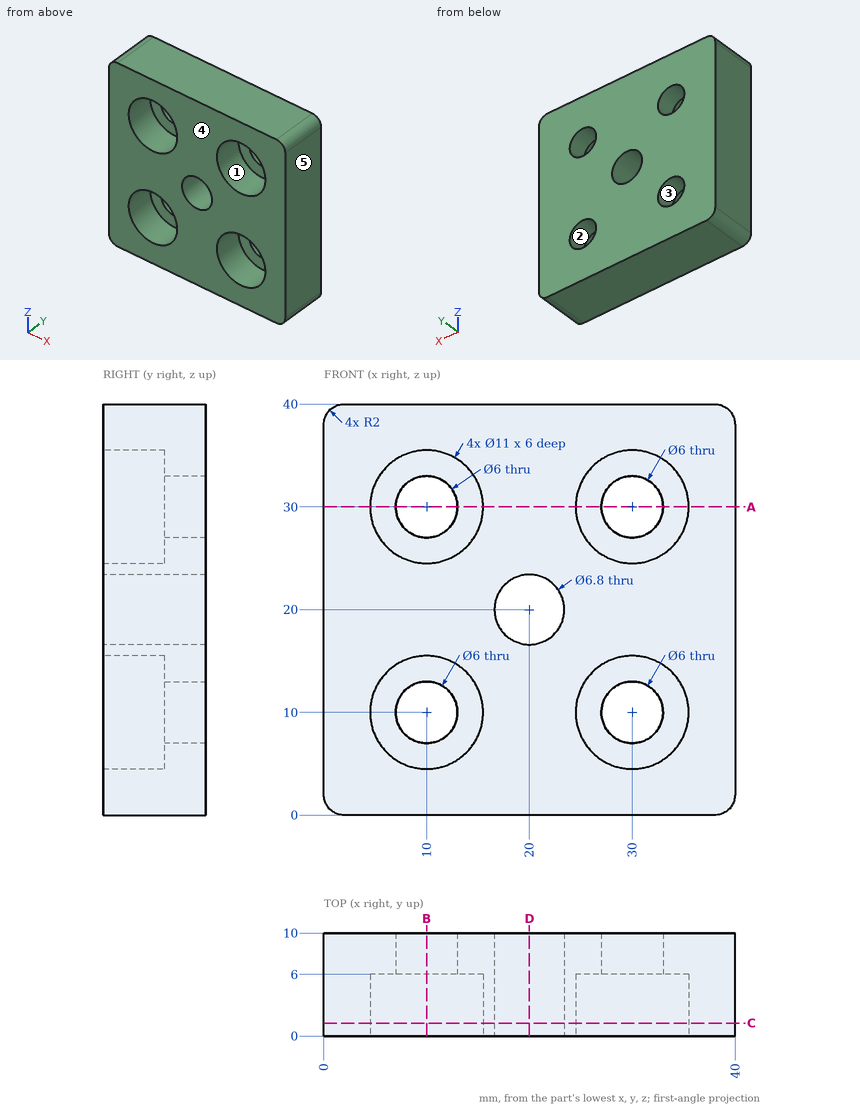
Here's the drawing with two shaded views (mm, measured from the low corner). I have some questions. A direction names the side the tool comes from. Give positions to 0.01 mm unless a question says otherwise; leave off trailing zeros. Loops run counter-clockwise (first coordinate to the right, second up) from the corner with the lowest first, then second, coordinate; pieces in that order, holes last. Notation, with made-up numbers: (-5, 23) -> (12, 23) arc R24 ccw to (12, 62) -> close; hole circle Ø5 at (-36.75, 13). An arc over 180 degrees is marked (long way). One line per item, written item: value.
Q1. Suppose I cut it at A-A on z = 30. Please give me the cut outline in (x, y).
Answers follow:
outline: (0, 0) -> (4.5, 0) -> (4.5, 6) -> (7, 6) -> (7, 10) -> (0, 10) -> close; (13, 6) -> (15.5, 6) -> (15.5, 0) -> (24.5, 0) -> (24.5, 6) -> (27, 6) -> (27, 10) -> (13, 10) -> close; (33, 6) -> (35.5, 6) -> (35.5, 0) -> (40, 0) -> (40, 10) -> (33, 10) -> close
Q2. Suppose I cut it at D-D on x = 20. Please give me the cut outline in (y, z), then the cut area to 3 significant figures.
Answers follow:
outline: (0, 0) -> (10, 0) -> (10, 16.6) -> (0, 16.6) -> close; (0, 23.4) -> (10, 23.4) -> (10, 40) -> (0, 40) -> close
area: 332 mm^2
Q3. Suppose I cut it at C-C on y = 1.25. Please give me the cut outline in (x, z).
Answers follow:
outline: (0, 2) arc R2 ccw to (2, 0) -> (38, 0) arc R2 ccw to (40, 2) -> (40, 38) arc R2 ccw to (38, 40) -> (2, 40) arc R2 ccw to (0, 38) -> close; hole circle Ø11 at (10, 10); hole circle Ø11 at (10, 30); hole circle Ø6.8 at (20, 20); hole circle Ø11 at (30, 10); hole circle Ø11 at (30, 30)
Q4. We'd pull the mould along X, two halves only. Please class the marked faces 3, 4 and 5: pulls with the +X half, pulls with the -X half, needs draft (parallel to the pull), parting line crosses it, or undercut.
Answers follow:
face 3: undercut
face 4: needs draft
face 5: pulls with the +X half
Q5. If I drill on line 1 along X through (y, z) = (6.95, 30); line 2 along X through (y, z) = (4.8, 10), over which ranges is the centre line in solid material (lowest first)?
Answers follow:
line 1: 0 to 7, 13 to 27, 33 to 40
line 2: 0 to 4.5, 15.5 to 24.5, 35.5 to 40
Q6. Suppose I cut it at B-B on x = 10. Please give me the cut outline in (y, z), then the cut area to 3 significant figures.
Answers follow:
outline: (0, 0) -> (10, 0) -> (10, 7) -> (6, 7) -> (6, 4.5) -> (0, 4.5) -> close; (0, 15.5) -> (6, 15.5) -> (6, 13) -> (10, 13) -> (10, 27) -> (6, 27) -> (6, 24.5) -> (0, 24.5) -> close; (0, 35.5) -> (6, 35.5) -> (6, 33) -> (10, 33) -> (10, 40) -> (0, 40) -> close
area: 220 mm^2
Q7. On a 3-axis mill with a long thin cutter (end or side, diameter ignored), from which of +Z, -Z, +X, -X, +Y, -Y can I reach the whole of each face in a straight line? I mean the marked faces 1 and 2. Say none if no direction works.
Answers follow:
face 1: -Y
face 2: +Y, -Y
Q8. I'm going to push flat-ended pins straight in: pin 1 Ø17.5 at (x, z) = (10, 10) entering from +Y; pin 2 Ø3.5 at (x, z) = (10, 12.5) entering from -Y. Where does each tip first touch, or does it pass through?
Answers follow:
pin 1: y = 10
pin 2: y = 6
